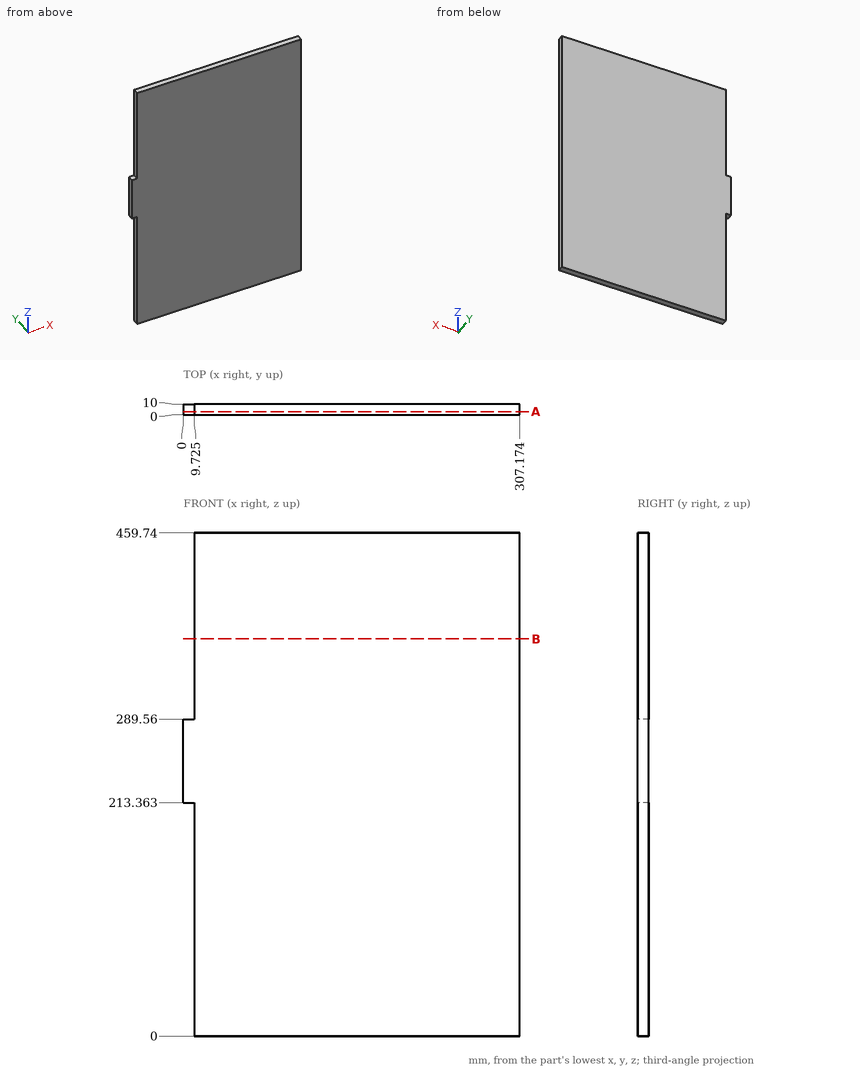
Design review of the part shown in the three views and the two pictorial views. Dimensions are in mm from the part's minimum x, y and z. Round coordinates to 2 decimals unless told otherwise and drop trailing zeros. Write each loop counter-clockwise with the first axis right and the second up, starting at its lowest first coordinate (ties: lowest second). Pieces come first, ordered by that corner, then holes.
Item 1: Consider section B-B on z = 363. Give the boundary of the cut face in (x, y) (1 decimal).
Item 2: Consider section A-A on y = 3. Give the boundary of the cut face in (x, z) (1 decimal).
Item 3: For pin 1 Ø2 at (x, z) = (151.5, 238) entering from -Y; pin 2 Ø5 at (y, z) = (2, 160) entering from -X (1 decimal); pin 3 Ø3 at (x, y) = (6, 4) entering from -Z, all flat-tipped, find the tip position at first contact; note any pin that passes through.
Item 4: Wall thickness on L1, parallel to X at y = 6.25, z = 178.5 (1 decimal): over which ranges is the line inside the solid? List them lowest first.
Check values:
1. outline: (9.7, 0) - (307.2, 0) - (307.2, 10) - (9.7, 10) - close
2. outline: (0, 213.4) - (9.7, 213.4) - (9.7, 0) - (307.2, 0) - (307.2, 459.7) - (9.7, 459.7) - (9.7, 289.6) - (0, 289.6) - close
3. pin 1: stops at y = 0
3. pin 2: stops at x = 9.7
3. pin 3: stops at z = 213.36
4. L1: x = 9.7 to 307.2
